Source: CAD feature listing. Evaluate the final solid. Frame: model axes, mm. Face numbers are marked on the shaded views. A direction names the side the tool comes from. Give positions to 0.01 mm unless a question says otherwise; leave off trailing zeros. Order: outer loops, then holes, each group sorted by start corner. A loop starts at its lowest first (then second) coordinate and runs counter-clockwise, first axis right, second up. Notation, with made-up numbers: (-13.5, 44.25) - (33.5, 44.25) arc R28 ccw to (33.5, 62.25) - close; hole circle Ø6 at (37.25, 10.25). An arc over 180 degrees is marked (long way). Use CSV: the item, a comma, the result in double quotes.
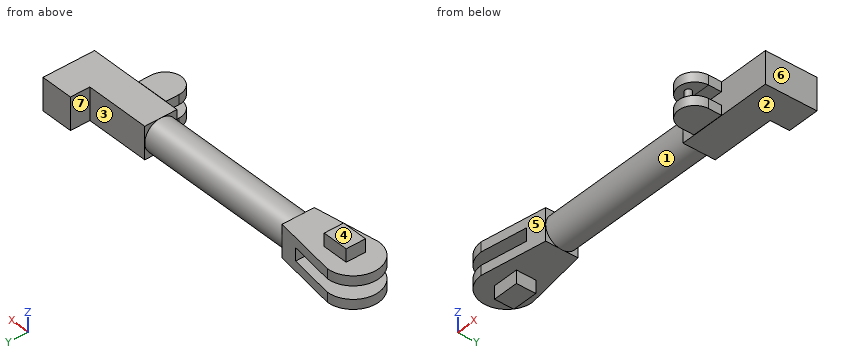
```python
from build123d import *

# Parameters (mm, degrees)
BOSS_EXTRUDE2_DEPTH  = 127
SKETCH11_W           = 279.4
SKETCH11_H           = 50.8
CUT_EXTRUDE1_DEPTH   = 350.192267956
SKETCH12_R           = 63.5
BOSS_EXTRUDE3_DEPTH  = 635
SKETCH13_W           = 101.6
SKETCH13_H           = 76.2
BOSS_EXTRUDE4_DEPTH  = 50.8
SKETCH14_W           = 127
SKETCH14_H           = 127
BOSS_EXTRUDE6_DEPTH  = 254
SKETCH15_W           = 127
SKETCH15_H           = 203.2
BOSS_EXTRUDE7_DEPTH  = 127
SKETCH16_W           = 127
SKETCH16_H           = 50.8
BOSS_EXTRUDE9_DEPTH  = 63.5
BOSS_EXTRUDE10_DEPTH = 38.1
SKETCH21_R           = 12.7
BOSS_EXTRUDE11_DEPTH = 50.8
SKETCH22_R           = 12.7
BOSS_EXTRUDE12_DEPTH = 50.8
SKETCH24_W           = 50.922560847
SKETCH24_H           = 50.8
CUT_EXTRUDE2_DEPTH   = 271.018


with BuildPart() as part:
    # Sketch9 → Boss-Extrude2 (new body)
    with BuildSketch(Plane.XY):
        with BuildLine():
            Line((0, 101.6), (254, 63.5))
            Line((254, 63.5), (254, 0))
            Line((254, 0), (254, -63.5))
            Line((254, -63.5), (0, -101.6))
            ThreePointArc((0, -101.6), (-101.6, 0), (0, 101.6))
        make_face()
    extrude(amount=BOSS_EXTRUDE2_DEPTH)

    # Sketch11 → Cut-Extrude1 (cut, through all)
    with BuildSketch(Plane(origin=(0, 101.6, 0), x_dir=(1, 0, 0), z_dir=(0, 1, 0))):
        with Locations((38.1, -63.5)):
            Rectangle(SKETCH11_W, SKETCH11_H)
    extrude(amount=-CUT_EXTRUDE1_DEPTH, mode=Mode.SUBTRACT)

    # Sketch12 → Boss-Extrude3 (add)
    with BuildSketch(Plane(origin=(254, 0, 0), x_dir=(0, 0, -1), z_dir=(1, 0, 0))):
        with Locations(Location((-62.280099892, 0, 0), (0, 0, 90))):
            Circle(SKETCH12_R)
    extrude(amount=BOSS_EXTRUDE3_DEPTH)

    # Sketch13 → Boss-Extrude4 (add)
    with BuildSketch(Plane.XY.offset(127)):
        with Locations((38.1, 0)):
            Rectangle(SKETCH13_W, SKETCH13_H)
    boss_extrude4 = extrude(amount=BOSS_EXTRUDE4_DEPTH)

    # Mirror1: Boss-Extrude4 across plane
    add(boss_extrude4.mirror(Plane.XY.offset(63.5)))

    # Sketch14 → Boss-Extrude6 (add)
    with BuildSketch(Plane(origin=(889, 0, 0), x_dir=(0, 0, -1), z_dir=(1, 0, 0))):
        with Locations((-62.280099892, 0)):
            Rectangle(SKETCH14_W, SKETCH14_H)
    extrude(amount=BOSS_EXTRUDE6_DEPTH)

    # Sketch15 → Boss-Extrude7 (add)
    with BuildSketch(Plane(origin=(1143, 0, 0), x_dir=(0, 0, -1), z_dir=(1, 0, 0))):
        with Locations((-62.280099892, 38.1)):
            Rectangle(SKETCH15_W, SKETCH15_H)
    extrude(amount=BOSS_EXTRUDE7_DEPTH)

    # Sketch16 → Boss-Extrude9 (add)
    with BuildSketch(Plane.XY.offset(63.5)):
        with Locations((1003.3, -88.9)):
            Rectangle(SKETCH16_W, SKETCH16_H)
    boss_extrude9 = extrude(amount=BOSS_EXTRUDE9_DEPTH)

    # Sketch20 → Boss-Extrude10 (add)
    with BuildSketch(Plane.XY.offset(127)):
        with BuildLine():
            Line((939.8, -114.3), (1066.8, -114.3))
            ThreePointArc((1066.8, -114.3), (1003.3, -177.8), (939.8, -114.3))
        make_face()
    boss_extrude10 = extrude(amount=-BOSS_EXTRUDE10_DEPTH)

    # Mirror2: Boss-Extrude9, Boss-Extrude10 across plane
    add(boss_extrude9.mirror(Plane.XY.offset(63.5)))
    add(boss_extrude10.mirror(Plane.XY.offset(63.5)))

    # Sketch21 → Boss-Extrude11 (add)
    with BuildSketch(Plane.XY.offset(38.1)):
        with Locations(Location((0, 0, 0), (0, 0, 180))):
            Circle(SKETCH21_R)
    extrude(amount=BOSS_EXTRUDE11_DEPTH)

    # Sketch22 → Boss-Extrude12 (add)
    with BuildSketch(Plane.XY.offset(38.1)):
        with Locations(Location((1003.3, -139.7, 0), (0, 0, 180))):
            Circle(SKETCH22_R)
    extrude(amount=BOSS_EXTRUDE12_DEPTH)

    # Sketch24 → Cut-Extrude2 (cut)
    with BuildSketch(Plane(origin=(1066.8, 0, 0), x_dir=(0, 0, -1), z_dir=(1, 0, 0))):
        with Locations((-63.561280424, -88.9)):
            Rectangle(SKETCH24_W, SKETCH24_H)
    extrude(amount=-CUT_EXTRUDE2_DEPTH, mode=Mode.SUBTRACT)


solid = part.part
```
Item 1: Section A-A on x = 1003.3. Return the cut outline in (y, z).
Filled in:
outline,"(-177.8, 0) - (-63.5, 0) - (-63.5, -1.22) - (63.5, -1.22) - (63.5, 125.78) - (-63.5, 125.78) - (-63.5, 127) - (-177.8, 127) - (-177.8, 88.9) - (-152.4, 88.9) - (-152.4, 38.1) - (-177.8, 38.1) - close; hole (-127, 38.1) - (-63.5, 38.1) - (-63.5, 89.02) - (-114.3, 89.02) - (-114.3, 88.9) - (-127, 88.9) - close"
Item 2: Mould query, pull axis X, two halves, no side actions, for the marked faces 4, 5, 6 and 7. Classes: released by +X, released by -X, zero draft, split by the parting line, or undercut.
Filled in:
face 4,"zero draft"
face 5,"undercut"
face 6,"released by +X"
face 7,"undercut"
Item 3: Material intervals for line 1 (Z direction, x = 1189, y = 59); line 2 (Y direction, x = 1070, z = 8); line 3 (X direction, y = 116.5, z = 46.5), sorted ascending. Write a range as from..to.
Filled in:
line 1,"z = -1.22..125.78"
line 2,"y = -63.5..63.5"
line 3,"x = 1143..1270"
Item 4: Section B-B on x = 140.5. Return the cut outline in (y, z) (3 decimals).
Filled in:
outline,"(-80.525, 0) - (80.525, 0) - (80.525, 38.1) - (-80.525, 38.1) - close; (-80.525, 88.9) - (80.525, 88.9) - (80.525, 127) - (-80.525, 127) - close"
Item 5: Section D-D on x = 588.5. Return the cut outline in (y, z).
Filled in:
outline,"circle Ø127 at (0, 62.28)"
Item 6: First-contact query: pin 1 (12 mm diameter, centred on x = 207.5, z = 44, fed in from +Y) (3 decimals); pin 2 (1.5 mm diameter, centred on x = 796.5, z = 15, fed in from -Y); pin 3 (1.5 mm diameter, centred on x = 1093.5, z = 48.5, fed in from +Y). Flat tips, straight axial feed; report the tip coordinate or a pass-through.
Filled in:
pin 1,"stops at y = 71.375"
pin 2,"stops at y = -43.21"
pin 3,"stops at y = 63.5"
Item 7: Set-up query: the marked faces 1, 2 and 3. Return all of +Z, -Z, +X, -X, +Y, -Y with unobstructed straight access to the full face (end or side cutting, diameter ignored); none if empty.
Filled in:
face 1,"none"
face 2,"-Z, +X, +Y, -Y"
face 3,"+Z, -Z, +Y"
Item 8: Section C-C on y = -139.7. Return the cut outline in (x, z), then the cut area to 3 significant figures.
Filled in:
outline,"(945.1, 0) - (1061.5, 0) - (1061.5, 38.1) - (1016, 38.1) - (1016, 88.9) - (1061.5, 88.9) - (1061.5, 127) - (945.1, 127) - (945.1, 88.9) - (990.6, 88.9) - (990.6, 38.1) - (945.1, 38.1) - close"
area,"10,200 mm2"
